```python
from build123d import *

# Parameters (mm, degrees)
SKETCH1_W             = 5
SKETCH1_H             = 69.5
BOSS_EXTRUDE1_DEPTH   = 30
BOSS_EXTRUDE1_2_DEPTH = 30
SKETCH1_4_W           = 67
SKETCH1_4_H           = 69.5
BOSS_EXTRUDE3_DEPTH   = 5
SKETCH2_R             = 6.477
CUT_EXTRUDE1_DEPTH    = 34
SKETCH3_R             = 4
CUT_EXTRUDE2_DEPTH    = 119
CUT_EXTRUDE3_DEPTH    = 14
SKETCH9_W             = 19.710117916
SKETCH9_H             = 20.225929664
CUT_EXTRUDE4_DEPTH    = 113
FILLET1_R             = 10
FILLET2_R             = 4
SKETCH11_R            = 2.4003
CUT_EXTRUDE5_DEPTH    = 5


with BuildPart() as part:
    # Sketch1 → Boss-Extrude1 (new body)
    with BuildSketch(Plane(origin=(0, 0, 0), x_dir=(1, 0, 0), z_dir=(0, 1, 0))):
        with Locations((-36, 0)):
            Rectangle(SKETCH1_W, SKETCH1_H)
    extrude(amount=BOSS_EXTRUDE1_DEPTH)



with BuildPart() as body_2:
    # Sketch1 → Boss-Extrude1 2 (new body)
    with BuildSketch(Plane(origin=(0, 0, 0), x_dir=(1, 0, 0), z_dir=(0, 1, 0))):
        with Locations((36, 0)):
            Rectangle(SKETCH1_W, SKETCH1_H)
    extrude(amount=BOSS_EXTRUDE1_2_DEPTH)


with BuildPart() as part_1:
    add(part.part)

    add(body_2.part)  # Boss-Extrude3 merges body 2
    # Sketch1<4> → Boss-Extrude3 (add)
    with BuildSketch(Plane(origin=(0, 0, 0), x_dir=(1, 0, 0), z_dir=(0, 1, 0))):
        Rectangle(SKETCH1_4_W, SKETCH1_4_H)
    extrude(amount=BOSS_EXTRUDE3_DEPTH)

    # Sketch2 → Cut-Extrude1 (cut)
    with BuildSketch(Plane.ZY.offset(38.5)):
        with Locations((0, 17.124630649)):
            Circle(SKETCH2_R)
    extrude(amount=-CUT_EXTRUDE1_DEPTH, mode=Mode.SUBTRACT)

    # Sketch3 → Cut-Extrude2 (cut)
    with BuildSketch(Plane(origin=(0, 5, 0), x_dir=(1, 0, 0), z_dir=(0, 1, 0))):
        with Locations((-22.5, 26)):
            Circle(SKETCH3_R)
        with Locations((-22.5, -26)):
            Circle(SKETCH3_R)
        with Locations((22.5, 26)):
            Circle(SKETCH3_R)
        with Locations((22.5, -26)):
            Circle(SKETCH3_R)
    extrude(amount=-CUT_EXTRUDE2_DEPTH, mode=Mode.SUBTRACT)

    # Sketch8 → Cut-Extrude3 (cut)
    with BuildSketch(Plane(origin=(38.5, 0, 0), x_dir=(0, 0, -1), z_dir=(1, 0, 0))):
        with BuildLine():
            Line((-1.524, 19.156630649), (1.524, 19.156630649))
            ThreePointArc((1.524, 19.156630649), (0, 14.584630649), (-1.524, 19.156630649))
        make_face()
    extrude(amount=-CUT_EXTRUDE3_DEPTH, mode=Mode.SUBTRACT)

    # Sketch9 → Cut-Extrude4 (cut)
    with BuildSketch(Plane.ZY.offset(38.5)):
        with Locations((-24.894941042, 19.887035168)):
            Rectangle(SKETCH9_W, SKETCH9_H)
        with Locations((24.894941042, 19.887035168)):
            Rectangle(SKETCH9_W, SKETCH9_H)
    extrude(amount=-CUT_EXTRUDE4_DEPTH, mode=Mode.SUBTRACT)

    # Fillet1
    fillet1_edges = [part_1.edges().sort_by_distance(p)[0] for p in [
        (36, 9.774070336, -15.039882084),
        (-36, 30, -15.039882084),
        (-36, 9.774070336, -15.039882084),
        (36, 9.774070336, 15.039882084),
        (-36, 9.774070336, 15.039882084),
        (-36, 30, 15.039882084),
        (36, 30, 15.039882084),
        (36, 30, -15.039882084),
    ]]
    fillet(fillet1_edges, radius=FILLET1_R)

    # Fillet2
    fillet2_edges = [part_1.edges().sort_by_distance(p)[0] for p in [
        (36, 9.774070336, -34.75),
        (-36, 9.774070336, -34.75),
        (36, 9.774070336, 34.75),
        (-36, 9.774070336, 34.75),
    ]]
    fillet(fillet2_edges, radius=FILLET2_R)

    # Sketch11 → Cut-Extrude5 (cut)
    with BuildSketch(Plane.ZY.offset(-33.5)):
        with Locations((-5.856308805, 22.980939454)):
            Circle(SKETCH11_R)
        with Locations((5.856308805, 22.980939454)):
            Circle(SKETCH11_R)
        with Locations((-5.856308805, 11.268321844)):
            Circle(SKETCH11_R)
        with Locations((5.856308805, 11.268321844)):
            Circle(SKETCH11_R)
    extrude(amount=-CUT_EXTRUDE5_DEPTH, mode=Mode.SUBTRACT)


solid = part_1.part
```
The model under review builds one solid part; all positions refer to its coordinate system, in mm. A direction names the side the tool comes from. Round coordinates to 2 decimals unless told otherwise and drop trailing zeros. Order: outer loops, then holes, each group sorted by start corner. A loop starts at its lowest first (then second) coordinate and runs counter-clockwise, first axis right, second up.
Item 1: Machinability: for faces 4 (the flat face through (36, 9.774, -28)), 5 (the flat face through (33.5, 12, 0)), 6 (the cylindrical face through (-36.035, 22.586, 3.482)), 7 (the cylindrical face through (35.965, 8.925, -6.377)), which of the approach directions +Z, -Z, +X, -X, +Y, -Y give a long, thin tool a straight path to every point of the face, cutting with its end or side? Answer none if there is none.
Working result:
face 4: -Z, +X, -X, +Y
face 5: +Z, -Z, +Y
face 6: -X
face 7: +X
Item 2: To check wall thickness, follow probe 1 along Z at (x, y) = (22.5, 2.7); probe 2 along X at (y, z) = (19.75, 11.5); probe 3 along X at (y, z) = (3.25, 28.5). State the ranges of each line that lie inside material, in increasing order.
Working result:
probe 1: z = -34.75 to -30, -22 to 22, 30 to 34.75
probe 2: x = -38.5 to -33.5, 33.5 to 38.5
probe 3: x = -38.5 to -25.62, -19.38 to 19.38, 25.62 to 38.5
Item 3: Draft analysis for pull direction Z (two halves, no side actions). For faces 1 (the cylindrical face through (-35.965, 12.626, -18.047)), 2 (the flat face through (0, 5, 0)), 3 (the cylindrical face through (19.55, 2.54, -28.7)), state which applies: released by +Z, released by -Z, zero draft, split by the parting line, or undercut.
Working result:
face 1: released by -Z
face 2: zero draft
face 3: undercut
Item 4: Add section C-C, the plane x = -22.5. State the section outline as (y, z) points, and give its area (4 significant figures).
Working result:
outline: (0, -34.75) - (5, -34.75) - (5, -30) - (0, -30) - close; (0, -22) - (5, -22) - (5, 22) - (0, 22) - close; (0, 30) - (5, 30) - (5, 34.75) - (0, 34.75) - close
area: 267.5 mm2
Item 5: Add section D-D, the plane z = 0. State the section outline as (x, y) points, and give its area (3 significant figures).
Working result:
outline: (-38.5, 0) - (38.5, 0) - (38.5, 14.58) - (33.5, 14.58) - (33.5, 5) - (-33.5, 5) - (-33.5, 10.65) - (-38.5, 10.65) - close; (-38.5, 23.6) - (-33.5, 23.6) - (-33.5, 30) - (-38.5, 30) - close; (33.5, 19.16) - (38.5, 19.16) - (38.5, 30) - (33.5, 30) - close
area: 547 mm2
Item 6: Add section B-B, the plane z = 26. State the section outline as (x, y) points, and give its area (3 significant figures).
Working result:
outline: (-38.5, 0) - (-26.5, 0) - (-26.5, 5) - (-33.5, 5) - (-33.5, 9.77) - (-38.5, 9.77) - close; (-18.5, 0) - (18.5, 0) - (18.5, 5) - (-18.5, 5) - close; (26.5, 0) - (38.5, 0) - (38.5, 9.77) - (33.5, 9.77) - (33.5, 5) - (26.5, 5) - close
area: 353 mm2
Item 7: For pin 1 (5.5 mm diameter, centred on x = -37, z = 29, fed in from +Y); pin 2 (6 mm diameter, centred on x = -21.5, z = -16, fed in from +Y); pin 3 (4 mm diameter, centred on y = 22.98, z = -5.86, fed in from +X), all flat-tipped, find the tip position at first contact; note any pin that passes through.
Working result:
pin 1: stops at y = 9.77
pin 2: stops at y = 5
pin 3: stops at x = -33.5
Item 8: Add section A-A, the plane y = 3.5. State the section outline as (x, z) points.
Working result:
outline: (-38.5, -34.75) - (38.5, -34.75) - (38.5, 34.75) - (-38.5, 34.75) - close; hole circle Ø8 at (-22.5, -26); hole circle Ø8 at (-22.5, 26); hole circle Ø8 at (22.5, -26); hole circle Ø8 at (22.5, 26)
